Here's how the part is built. I have some questions about the finished solid (model axes, mm). Give positions to 0.01 mm unless a question says otherwise; leave off trailing zeros. Order: outer loops, then holes, each group sorted by start corner. A loop starts at its lowest first (then second) coordinate and runs counter-clockwise, first axis right, second up. Notation, with made-up numbers: (34, -24) - (60, -24) arc R33 ccw to (60, 12) - close; hole circle Ø10 at (-22, 15). An arc over 180 degrees is marked (long way). One line per question, with ' | ' between items.
from build123d import *

# Parameters (mm, degrees)
SKETCH1_R           = 100
SKETCH1_R_2         = 25
BOSS_EXTRUDE1_DEPTH = 6
SKETCH2_R           = 1.6
CUT_EXTRUDE1_DEPTH  = 142.548578234


with BuildPart() as part:
    # Sketch1 → Boss-Extrude1 (new body)
    with BuildSketch(Plane.XY):
        Circle(SKETCH1_R)
        Circle(SKETCH1_R_2, mode=Mode.SUBTRACT)
    extrude(amount=BOSS_EXTRUDE1_DEPTH)

    # Sketch2 → Cut-Extrude1 (cut, through all)
    with BuildSketch(Plane(origin=(0, 0, 0), x_dir=(-1, 0, 0), z_dir=(0, 0, -1))):
        with Locations((-16.129709466, 32)):
            Circle(SKETCH2_R)
        with Locations((13.870290534, 32)):
            Circle(SKETCH2_R)
        with Locations(Location((13.870290534, -32, 0), (0, 0, 180))):
            Circle(SKETCH2_R)
        with Locations(Location((-16.129709466, -32, 0), (0, 0, 180))):
            Circle(SKETCH2_R)
    extrude(amount=-CUT_EXTRUDE1_DEPTH, mode=Mode.SUBTRACT)


solid = part.part
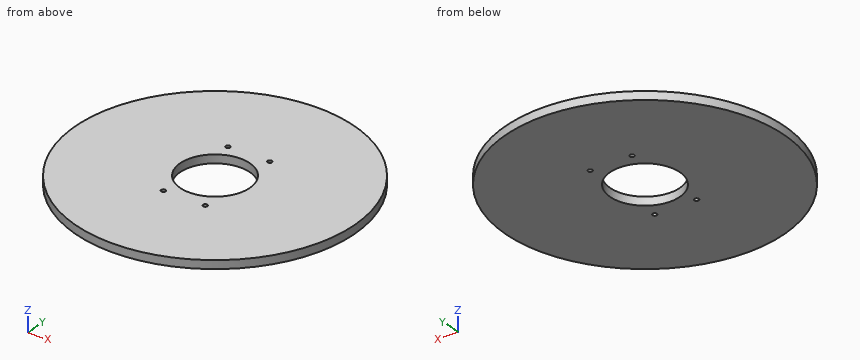
1) I'm going to push flat-ended pins straight in: P1, Ø1.9, axis at x = 16.13, y = 32, coming from the +Z side; P2, Ø1, axis at y = -56.5, z = 1, coming from the -X side; P3, Ø3, axis at y = 43.5, z = 3.5, coming from the -X side; P4, Ø2, axis at y = 17.5, z = 3, coming from the +X side. Where does each tip first touch, or does it pass through?
Model answer:
P1: passes through | P2: stops at x = -82.85 | P3: stops at x = -90.75 | P4: stops at x = 98.63
2) I want a section at C-C (z = 4.45). List the corners of the cut face in (x, y) for me, plus the area to 3 significant figures.
Model answer:
outline: circle Ø200 at (0, 0); hole circle Ø50 at (0, 0); hole circle Ø3.2 at (-13.87, -32); hole circle Ø3.2 at (-13.87, 32); hole circle Ø3.2 at (16.13, -32); hole circle Ø3.2 at (16.13, 32) | area: 29,400 mm2
3) I want a section at A-A (x = 0). List the corners of the cut face in (y, z) for me.
Model answer:
outline: (-100, 0) - (-25, 0) - (-25, 6) - (-100, 6) - close; (25, 0) - (100, 0) - (100, 6) - (25, 6) - close
4) I want a section at D-D (x = -79.5). List the corners of the cut face in (y, z) for me.
Model answer:
outline: (-60.66, 0) - (60.66, 0) - (60.66, 6) - (-60.66, 6) - close
5) Please list where these lines run through material, in increasing order: L1, parallel to X at y = -5.5, z = 3.7; L2, parallel to X at y = -19.5, z = 4.6; L3, parallel to Y at x = 20, z = 1.45.
Model answer:
L1: x = -99.85 to -24.39, 24.39 to 99.85 | L2: x = -98.08 to -15.64, 15.64 to 98.08 | L3: y = -97.98 to -15, 15 to 97.98
